Input: part model. Units: mm. Frame: model coordinates. A direction names the side the tool comes from. Coordinates: 2 decimals unless noted, no trailing zeros. Write each loop counter-clockwise with the first axis right and the second up, starting at its lowest first coordinate (ties: lowest second). Pieces come first, ordered by that corner, then holes. Notation, with made-up numbers: M 11,35 L 55,35 A27 cw 55,53 Z; hole C -9,15.5 d4. An arc over 180 degrees is marked long. Use one line per item in the form item = value.
from build123d import *
from build123d.topology import SkipClean

# Parameters (mm, degrees)
BOSS_EXTRUDE1_DEPTH = 31
BOSS_EXTRUDE3_DEPTH = 10
BOSS_EXTRUDE4_DEPTH = 5
SKETCH6_W           = 19
SKETCH6_H           = 10.5
SKETCH6_R           = 2.25
SKETCH6_W_2         = 50
SKETCH6_W_3         = 96
CUT_EXTRUDE1_DEPTH  = 94.490641243
CUT_EXTRUDE2_DEPTH  = 10
SKETCH9_W           = 96
SKETCH9_H           = 4
SKETCH9_W_2         = 19
SKETCH9_W_3         = 50
CUT_EXTRUDE4_DEPTH  = 20
BOSS_EXTRUDE5_DEPTH = 31
FILLET3_R           = 5


with BuildPart() as part:
    # Sketch1 → Boss-Extrude1 (new body)
    with BuildSketch(Plane.XY):
        with BuildLine():
            ThreePointArc((-50.477717856, -31.5), (-51.659400485, -29.522133079), (-52.763623833, -27.5))
            Line((-52.763623833, -27.5), (-57.236352085, -27.5))
            ThreePointArc((-57.236352085, -27.5), (0, -63.5), (57.236352085, -27.5))
            Line((57.236352085, -27.5), (52.763623833, -27.5))
            ThreePointArc((52.763623833, -27.5), (51.659400485, -29.522133079), (50.477717856, -31.5))
            ThreePointArc((50.477717856, -31.5), (49.272860314, -33.353189299), (48, -35.160346983))
            ThreePointArc((48, -35.160346983), (0, -59.5), (-48, -35.160346983))
            ThreePointArc((-48, -35.160346983), (-49.272860314, -33.353189299), (-50.477717856, -31.5))
        make_face()
        with BuildLine():
            Line((52.763623833, -27.5), (-52.763623833, -27.5))
            ThreePointArc((-52.763623833, -27.5), (-51.659400485, -29.522133079), (-50.477717856, -31.5))
            Line((-50.477717856, -31.5), (-48, -31.5))
            Line((-48, -31.5), (48, -31.5))
            Line((48, -31.5), (50.477717856, -31.5))
            ThreePointArc((50.477717856, -31.5), (51.659400485, -29.522133079), (52.763623833, -27.5))
        make_face()
        with BuildLine():
            ThreePointArc((-56.868268832, 17.5), (-57.443088433, 15.50940332), (-57.948252778, 13.5))
            Line((-57.948252778, 13.5), (57.948252778, 13.5))
            ThreePointArc((57.948252778, 13.5), (57.443088433, 15.50940332), (56.868268832, 17.5))
            Line((56.868268832, 17.5), (52, 17.5))
            Line((52, 17.5), (48, 17.5))
            Line((48, 17.5), (-48, 17.5))
            Line((-48, 17.5), (-52, 17.5))
            Line((-52, 17.5), (-56.868268832, 17.5))
        make_face()
        with BuildLine():
            Line((-52, 28.917987482), (-52, 17.5))
            Line((-52, 17.5), (-48, 17.5))
            Line((-48, 17.5), (-48, 35.160346983))
            ThreePointArc((-48, 35.160346983), (-50.097322913, 32.101530134), (-52, 28.917987482))
        make_face()
        with BuildLine():
            Line((-62.04836823, 13.5), (-57.948252778, 13.5))
            ThreePointArc((-57.948252778, 13.5), (-57.443088433, 15.50940332), (-56.868268832, 17.5))
            ThreePointArc((-56.868268832, 17.5), (-54.732692234, 23.336289354), (-52, 28.917987482))
            ThreePointArc((-52, 28.917987482), (-50.097322913, 32.101530134), (-48, 35.160346983))
            Line((-48, 35.160346983), (-48, 41.572226306))
            ThreePointArc((-48, 41.572226306), (-56.78620704, 28.417893835), (-62.04836823, 13.5))
        make_face()
        with BuildLine():
            ThreePointArc((56.868268832, 17.5), (57.443088433, 15.50940332), (57.948252778, 13.5))
            Line((57.948252778, 13.5), (62.04836823, 13.5))
            ThreePointArc((62.04836823, 13.5), (56.78620704, 28.417893835), (48, 41.572226306))
            Line((48, 41.572226306), (48, 35.160346983))
            ThreePointArc((48, 35.160346983), (50.097322913, 32.101530134), (52, 28.917987482))
            ThreePointArc((52, 28.917987482), (54.732692234, 23.336289354), (56.868268832, 17.5))
        make_face()
        with BuildLine():
            Line((48, 17.5), (52, 17.5))
            Line((52, 17.5), (52, 28.917987482))
            ThreePointArc((52, 28.917987482), (50.097322913, 32.101530134), (48, 35.160346983))
            Line((48, 35.160346983), (48, 17.5))
        make_face()
        with BuildLine():
            ThreePointArc((44.294469181, 45.5), (0, 63.5), (-44.294469181, 45.5))
            Line((-44.294469181, 45.5), (-38.340579025, 45.5))
            ThreePointArc((-38.340579025, 45.5), (-35.733876731, 47.574573606), (-33.015148038, 49.5))
            ThreePointArc((-33.015148038, 49.5), (0, 59.5), (33.015148038, 49.5))
            ThreePointArc((33.015148038, 49.5), (35.733876731, 47.574573606), (38.340579025, 45.5))
            Line((38.340579025, 45.5), (44.294469181, 45.5))
        make_face()
        with BuildLine():
            ThreePointArc((-33.015148038, 49.5), (-35.733876731, 47.574573606), (-38.340579025, 45.5))
            Line((-38.340579025, 45.5), (38.340579025, 45.5))
            ThreePointArc((38.340579025, 45.5), (35.733876731, 47.574573606), (33.015148038, 49.5))
            Line((33.015148038, 49.5), (-33.015148038, 49.5))
        make_face()
        with BuildLine():
            ThreePointArc((48, -35.160346983), (49.272860314, -33.353189299), (50.477717856, -31.5))
            Line((50.477717856, -31.5), (48, -31.5))
            Line((48, -31.5), (48, -35.160346983))
        make_face()
        with BuildLine():
            Line((-48, -31.5), (-50.477717856, -31.5))
            ThreePointArc((-50.477717856, -31.5), (-49.272860314, -33.353189299), (-48, -35.160346983))
            Line((-48, -35.160346983), (-48, -31.5))
        make_face()
    extrude(amount=BOSS_EXTRUDE1_DEPTH)

    # Sketch2 → Boss-Extrude3 (add)
    with SkipClean():  # the faces are left unmerged after this step: merging them gives an invalid solid
        with BuildSketch(Plane(origin=(0, 0, 0), x_dir=(-1, 0, 0), z_dir=(0, 0, -1))):
            with BuildLine():
                ThreePointArc((48, 41.572226306), (46.189004231, 43.575519367), (44.294469181, 45.5))
                Line((44.294469181, 45.5), (25, 45.5))
                Line((25, 45.5), (25, 17.5))
                Line((25, 17.5), (48, 17.5))
                Line((48, 17.5), (48, 41.572226306))
            make_face()
            with BuildLine():
                Line((-25, 45.5), (-44.294469181, 45.5))
                ThreePointArc((-44.294469181, 45.5), (-46.189004231, 43.575519367), (-48, 41.572226306))
                Line((-48, 41.572226306), (-48, 17.5))
                Line((-48, 17.5), (-25, 17.5))
                Line((-25, 17.5), (-25, 45.5))
            make_face()
        extrude(amount=-BOSS_EXTRUDE3_DEPTH)

    # Sketch4 → Boss-Extrude4 (add)
    with SkipClean():  # the faces are left unmerged after this step: merging them gives an invalid solid
        with BuildSketch(Plane(origin=(0, 0, 0), x_dir=(-1, 0, 0), z_dir=(0, 0, -1))):
            with BuildLine():
                Line((-57.236352085, -27.5), (57.236352085, -27.5))
                ThreePointArc((57.236352085, -27.5), (63.067116036, -7.401950746), (62.04836823, 13.5))
                Line((62.04836823, 13.5), (-62.04836823, 13.5))
                ThreePointArc((-62.04836823, 13.5), (-63.067116036, -7.401950746), (-57.236352085, -27.5))
            make_face()
        extrude(amount=-BOSS_EXTRUDE4_DEPTH)

    # Sketch6 → Cut-Extrude1 (cut, through all)
    with SkipClean():  # the faces are left unmerged after this step: merging them gives an invalid solid
        with BuildSketch(Plane.XY.offset(5)):
            with Locations((-38.5, 8.25)):
                Rectangle(SKETCH6_W, SKETCH6_H)
            with Locations((-47.5, -7)):
                Circle(SKETCH6_R)
            with Locations((0, 8.25)):
                Rectangle(SKETCH6_W_2, SKETCH6_H)
            with Locations((0, -22.25)):
                Rectangle(SKETCH6_W_3, SKETCH6_H)
            with Locations((38.5, 8.25)):
                Rectangle(SKETCH6_W, SKETCH6_H)
            with Locations((47.5, -7)):
                Circle(SKETCH6_R)
        extrude(amount=-CUT_EXTRUDE1_DEPTH, mode=Mode.SUBTRACT)

    # Sketch7 → Cut-Extrude2 (cut)
    with SkipClean():  # the faces are left unmerged after this step: merging them gives an invalid solid
        with BuildSketch(Plane(origin=(0, 0, 0), x_dir=(-1, 0, 0), z_dir=(0, 0, -1))):
            with BuildLine():
                Line((-29, 17.5), (-48, 17.5))
                Line((-48, 17.5), (-48, 35.160346983))
                ThreePointArc((-48, 35.160346983), (-43.478741964, 40.618333265), (-38.340579025, 45.5))
                Line((-38.340579025, 45.5), (-29, 45.5))
                Line((-29, 45.5), (-29, 17.5))
            make_face()
            with BuildLine():
                Line((29, 17.5), (48, 17.5))
                Line((48, 17.5), (48, 35.160346983))
                ThreePointArc((48, 35.160346983), (43.478741964, 40.618333265), (38.340579025, 45.5))
                Line((38.340579025, 45.5), (29, 45.5))
                Line((29, 45.5), (29, 17.5))
            make_face()
        extrude(amount=-CUT_EXTRUDE2_DEPTH, mode=Mode.SUBTRACT)

    # Sketch9 → Cut-Extrude4 (cut)
    with SkipClean():  # the faces are left unmerged after this step: merging them gives an invalid solid
        with BuildSketch(Plane(origin=(0, 0, 0), x_dir=(-1, 0, 0), z_dir=(0, 0, -1))):
            with Locations((0, -29.5)):
                Rectangle(SKETCH9_W, SKETCH9_H)
            with Locations((-38.5, 15.5)):
                Rectangle(SKETCH9_W_2, SKETCH9_H)
            with Locations((0, 15.5)):
                Rectangle(SKETCH9_W_3, SKETCH9_H)
            with Locations((38.5, 15.5)):
                Rectangle(SKETCH9_W_2, SKETCH9_H)
            with Locations((0, 47.5)):
                Rectangle(SKETCH9_W_3, SKETCH9_H)
        extrude(amount=-CUT_EXTRUDE4_DEPTH, mode=Mode.SUBTRACT)

    # Sketch10 → Boss-Extrude5 (add)
    with SkipClean():  # the faces are left unmerged after this step: merging them gives an invalid solid
        with BuildSketch(Plane(origin=(0, 0, 0), x_dir=(-1, 0, 0), z_dir=(0, 0, -1))):
            with BuildLine():
                Line((-29.007574019, 51.950078436), (-29.007574019, 49.5))
                Line((-29.007574019, 49.5), (-25, 49.5))
                Line((-25, 49.5), (-25, 53.993055109))
                ThreePointArc((-25, 53.993055109), (-27.023100327, 53.009452447), (-29.007574019, 51.950078436))
            make_face()
            with BuildLine():
                ThreePointArc((29.007574019, 51.950078436), (27.023100327, 53.009452447), (25, 53.993055109))
                Line((25, 53.993055109), (25, 49.5))
                Line((25, 49.5), (29.007574019, 49.5))
                Line((29.007574019, 49.5), (29.007574019, 51.950078436))
            make_face()
        extrude(amount=-BOSS_EXTRUDE5_DEPTH)

    # Fillet3
    # the kernel refuses this fillet: 5 mm, written as the material it adds along each edge
    with BuildSketch(Plane(origin=(48, -17, 5), x_dir=(-1, 0, 0), z_dir=(0, 0, -1)), Plane(origin=(-48, -17, 5), x_dir=(0, -1, 0), z_dir=(0, 0, -1)), Plane(origin=(-29, 3, 5), x_dir=(0, 1, 0), z_dir=(0, 0, -1)), Plane(origin=(25, 3, 5), x_dir=(0, 1, 0), z_dir=(0, 0, -1)), Plane(origin=(48, 3, 5), x_dir=(0, 1, 0), z_dir=(0, 0, -1))) as fillet3_piece_1:
        with BuildLine():
            CenterArc((FILLET3_R, -FILLET3_R), FILLET3_R, 90, 90)
            Line((0, -FILLET3_R), (0, 0))
            Line((0, 0), (FILLET3_R, 0))
        make_face()
    extrude(amount=5)
    with BuildSketch(Plane(origin=(-48, 3, 5), x_dir=(0, 1, 0), z_dir=(0, 0, -1)), Plane(origin=(-25, 3, 5), x_dir=(0, 1, 0), z_dir=(0, 0, -1)), Plane(origin=(29, 3, 5), x_dir=(0, 1, 0), z_dir=(0, 0, -1))) as fillet3_piece_2:
        with BuildLine():
            CenterArc((FILLET3_R, FILLET3_R), FILLET3_R, 180, 90)
            Line((0, FILLET3_R), (0, 0))
            Line((0, 0), (FILLET3_R, 0))
        make_face()
    extrude(amount=5)
    with BuildSketch(Plane(origin=(48, -31.5, 20), x_dir=(0, 0, -1), z_dir=(0, 1, 0)), Plane(origin=(25, 49.5, 20), x_dir=(-1, 0, 0), z_dir=(0, -1, 0)), Plane(origin=(-29, 13.5, 20), x_dir=(0, 0, -1), z_dir=(0, 1, 0)), Plane(origin=(-48, 17.5, 20), x_dir=(0, 0, -1), z_dir=(0, -1, 0)), Plane(origin=(25, 13.5, 20), x_dir=(0, 0, -1), z_dir=(0, 1, 0))) as fillet3_piece_3:
        with BuildLine():
            CenterArc((FILLET3_R, FILLET3_R), FILLET3_R, 180, 90)
            Line((0, FILLET3_R), (0, 0))
            Line((0, 0), (FILLET3_R, 0))
        make_face()
    extrude(amount=4)
    with BuildSketch(Plane(origin=(-48, -27.5, 20), x_dir=(1, 0, 0), z_dir=(0, -1, 0)), Plane(origin=(-25, 45.5, 20), x_dir=(0, 0, -1), z_dir=(0, 1, 0)), Plane(origin=(-25, 17.5, 20), x_dir=(1, 0, 0), z_dir=(0, -1, 0)), Plane(origin=(48, 13.5, 20), x_dir=(-1, 0, 0), z_dir=(0, 1, 0)), Plane(origin=(29, 17.5, 20), x_dir=(1, 0, 0), z_dir=(0, -1, 0))) as fillet3_piece_4:
        with BuildLine():
            CenterArc((FILLET3_R, -FILLET3_R), FILLET3_R, 90, 90)
            Line((0, -FILLET3_R), (0, 0))
            Line((0, 0), (FILLET3_R, 0))
        make_face()
    extrude(amount=4)


solid = part.part
(1) Line query: probe 1 along Y at (x, z) = (-0.5, 22); probe 2 along Y at (x, z) = (12.5, 29.5); probe 3 along X at (y, z) = (9.5, 3). Output: solid intervals per line, ascending.
Computed:
probe_1 = -63.5 to -59.5, -31.5 to -27.5, 13.5 to 17.5, 45.5 to 49.5, 59.5 to 63.5
probe_2 = -62.26 to -58.17, -31.5 to -27.5, 13.5 to 17.5, 45.5 to 49.5, 58.17 to 62.26
probe_3 = -62.79 to -48, -29 to -25, 25 to 29, 48 to 62.79
(2) Pull-direction query (X, two-part tool) for faces 1 (the flat face through (-1, 49, 31)), 2 (the cylindrical face through (-46, 16, 19)); classes: pulls with the +X half, pulls with the -X half, needs draft (parallel to the pull), parting line crosses it, or undercut.
Computed:
face_1 = needs draft
face_2 = undercut
(3) First-contact query: pin 1 Ø4.5 at (x, z) = (31, 9) entering from +Y; pin 2 Ø16.5 at (y, z) = (23, 4) entering from -X; pin 3 Ø14.5 at (y, z) = (-27, 15.5) entering from -X. Flat tips, straight axial feed; report the tip coordinate or a pass-through.
Computed:
pin_1 = 56.62
pin_2 = -61.76
pin_3 = -57.24
(4) Section query B-B on x = -16. Return the cut outline in (y, z), plus the area to 3 significant figures.
Computed:
outline = M -61.45,0 L -57.31,0 L -57.31,31 L -61.45,31 Z; M -31.5,20 L -27.5,20 L -27.5,31 L -31.5,31 Z; M -17,0 L 3,0 L 3,5 L -17,5 Z; M 13.5,20 L 17.5,20 L 17.5,31 L 13.5,31 Z; M 45.5,20 L 49.5,20 L 49.5,31 L 45.5,31 Z; M 57.31,0 L 61.45,0 L 61.45,31 L 57.31,31 Z
area = 489 mm^2
(5) Section query D-D on y = -7. Return the cut outline in (x, z).
Computed:
outline = M -63.11,0 L -49.75,0 L -49.75,5 L -63.11,5 Z; M -45.25,0 L 45.25,0 L 45.25,5 L -45.25,5 Z; M 49.75,0 L 63.11,0 L 63.11,5 L 49.75,5 Z
(6) Section query A-A on z = 28.5. State how many separate pieces and enclosed holes the cut face has, plus the area to 3 significant figures.
Computed:
separate_pieces = 3
enclosed_holes = 6
area = 2,440 mm^2
(7) Set-up query: faces 3 (the flat face through (-25, 36, 9)), 4 (the cylindrical face through (24, 5, 3)), 5 (the flat face through (27, 32, 10)). Return all of +Z, -Z, +X, -X, +Y, -Y with unobstructed straight access to the full face (end or side cutting, diameter ignored); none if empty.
Computed:
face_3 = -Z
face_4 = +Z, -Z
face_5 = +Z
(8) Section query C-C on y = 55.5. Return the cut outline in (x, z), plus the area to 3 significant figures.
Computed:
outline = M -30.85,0 L -21.45,0 L -21.45,31 L -30.85,31 Z; M 21.45,0 L 30.85,0 L 30.85,31 L 21.45,31 Z
area = 583 mm^2
